Can you work these out from the model? Positions are in its coordinate system, mm. A direction names the side the tool comes from. Give positions to 0.01 mm unless a question says otherwise; leave off trailing zeros. Loops run counter-clockwise (first coordinate to the right, second up) from the corner with the lowest first, then second, coordinate; pieces in that order, holes last. Notation, with made-up numbers: (44.25, 35) -> (101.25, 35) arc R7 cw to (101.25, 46) -> close; hole circle Ø4 at (55, -11). An arc over 180 degrees is marked (long way). One line per question, with ' | ' between items.
from build123d import *

# Parameters (mm, degrees)
F0_W     = 101.6
F0_H     = 50.8
F1_DEPTH = 38.1


with BuildPart() as f1:
    # F0 (on Front) → F1 (new body, symmetric)
    with BuildSketch(Plane.XZ):
        with BuildLine():
            ThreePointArc((65.9712880145, -38.6489294899), (73.7903692418, -20.0232864477), (76.4588163197, 0))
            ThreePointArc((76.4588163197, 0), (73.9582301549, 19.3940915064), (66.6200350394, 37.5196151947))
            Line((66.6200350394, 37.5196151947), (65.9712880145, -38.6489294899))
        make_face()
        with BuildLine():
            Line((65.9712880145, -38.6489294899), (66.6200350394, 37.5196151947))
            ThreePointArc((66.6200350394, 37.5196151947), (66.5384735192, 37.6640695456), (66.4565987746, 37.808346596))
            Line((66.4565987746, 37.808346596), (0.8170776208, 76.4544503425))
            ThreePointArc((0.8170776208, 76.4544503425), (0.6511957232, 76.4560431695), (0.4853107601, 76.4572760859))
            Line((0.4853107601, 76.4572760859), (-65.8029574185, 38.9348351477))
            ThreePointArc((-65.8029574185, 38.9348351477), (-65.887277796, 38.7919736239), (-65.9712880145, 38.6489294899))
            Line((-65.9712880145, 38.6489294899), (-66.6200350394, -37.5196151947))
            ThreePointArc((-66.6200350394, -37.5196151947), (-66.5384735192, -37.6640695456), (-66.4565987746, -37.808346596))
            Line((-66.4565987746, -37.808346596), (-0.8170776208, -76.4544503425))
            ThreePointArc((-0.8170776208, -76.4544503425), (-0.6511957232, -76.4560431695), (-0.4853107601, -76.4572760859))
            Line((-0.4853107601, -76.4572760859), (65.8029574185, -38.9348351477))
            ThreePointArc((65.8029574185, -38.9348351477), (65.887277796, -38.7919736239), (65.9712880145, -38.6489294899))
        make_face()
        Rectangle(F0_W, F0_H, mode=Mode.SUBTRACT)
        with BuildLine():
            ThreePointArc((66.4565987746, 37.808346596), (66.5384735192, 37.6640695456), (66.6200350394, 37.5196151947))
            Line((66.6200350394, 37.5196151947), (66.6216664831, 37.7111608811))
            Line((66.6216664831, 37.7111608811), (66.4565987746, 37.808346596))
        make_face()
        with BuildLine():
            Line((65.9696565708, -38.8404751763), (65.9712880145, -38.6489294899))
            ThreePointArc((65.9712880145, -38.6489294899), (65.887277796, -38.7919736239), (65.8029574185, -38.9348351477))
            Line((65.8029574185, -38.9348351477), (65.9696565708, -38.8404751763))
        make_face()
        with BuildLine():
            Line((0.8170776208, 76.4544503425), (66.4565987746, 37.808346596))
            ThreePointArc((66.4565987746, 37.808346596), (38.7919736239, 65.887277796), (0.8170776208, 76.4544503425))
        make_face()
        with BuildLine():
            ThreePointArc((-0.4853107601, -76.4572760859), (37.6640695456, -66.5384735192), (65.8029574185, -38.9348351477))
            Line((65.8029574185, -38.9348351477), (-0.4853107601, -76.4572760859))
        make_face()
        with BuildLine():
            ThreePointArc((0.4853107601, 76.4572760859), (0.6511957232, 76.4560431695), (0.8170776208, 76.4544503425))
            Line((0.8170776208, 76.4544503425), (0.6520099123, 76.5516360573))
            Line((0.6520099123, 76.5516360573), (0.4853107601, 76.4572760859))
        make_face()
        with BuildLine():
            Line((-0.6520099123, -76.5516360573), (-0.4853107601, -76.4572760859))
            ThreePointArc((-0.4853107601, -76.4572760859), (-0.6511957232, -76.4560431695), (-0.8170776208, -76.4544503425))
            Line((-0.8170776208, -76.4544503425), (-0.6520099123, -76.5516360573))
        make_face()
        with BuildLine():
            Line((-65.8029574185, 38.9348351477), (0.4853107601, 76.4572760859))
            ThreePointArc((0.4853107601, 76.4572760859), (-37.6640695456, 66.5384735192), (-65.8029574185, 38.9348351477))
        make_face()
        with BuildLine():
            ThreePointArc((-66.4565987746, -37.808346596), (-38.7919736239, -65.887277796), (-0.8170776208, -76.4544503425))
            Line((-0.8170776208, -76.4544503425), (-66.4565987746, -37.808346596))
        make_face()
        with BuildLine():
            ThreePointArc((-65.9712880145, 38.6489294899), (-65.887277796, 38.7919736239), (-65.8029574185, 38.9348351477))
            Line((-65.8029574185, 38.9348351477), (-65.9696565708, 38.8404751763))
            Line((-65.9696565708, 38.8404751763), (-65.9712880145, 38.6489294899))
        make_face()
        with BuildLine():
            Line((-66.6216664831, -37.7111608811), (-66.4565987746, -37.808346596))
            ThreePointArc((-66.4565987746, -37.808346596), (-66.5384735192, -37.6640695456), (-66.6200350394, -37.5196151947))
            Line((-66.6200350394, -37.5196151947), (-66.6216664831, -37.7111608811))
        make_face()
        with BuildLine():
            Line((-66.6200350394, -37.5196151947), (-65.9712880145, 38.6489294899))
            ThreePointArc((-65.9712880145, 38.6489294899), (-76.4560431695, 0.6511957232), (-66.6200350394, -37.5196151947))
        make_face()
    extrude(amount=F1_DEPTH, both=True)


solid = f1.part
Q1. For pin 1 Ø10 at (y, z) = (14.5, -16.5) entering from +X; pin 2 Ø4 at (x, y) = (7, -15) entering from +Z; pin 3 Ø12 at (y, z) = (2.5, 5.5) entering from -X; pin 4 Ø6 at (x, y) = (-41.5, 28.5) entering from -Z, each with a flat end and sliding along its axis, tell me the tip position at first contact or that it passes through.
Entries:
pin 1: x = 75.59 | pin 2: z = 76.3 | pin 3: x = -76.46 | pin 4: z = -66.06
Q2. If we section it at C-C (z = -5): Write out the boundary of the cut face in (x, y).
Entries:
outline: (-76.3, -38.1) -> (-50.8, -38.1) -> (-50.8, 38.1) -> (-76.3, 38.1) -> close; (50.8, -38.1) -> (76.3, -38.1) -> (76.3, 38.1) -> (50.8, 38.1) -> close
Q3. If we section it at D-D (z = -27.5): Write out the boundary of the cut face in (x, y).
Entries:
outline: (-71.34, -38.1) -> (71.34, -38.1) -> (71.34, 38.1) -> (-71.34, 38.1) -> close
Q4. On a 3-axis mill with a long thin cutter (end or side, diameter ignored), from which of +Z, -Z, +X, -X, +Y, -Y can I reach the whole of each face in a straight line? I mean faces 1 (the face through (-1, -1, 25.4)), 2 (the face through (76.45, -0.53, -1.21)). Say none if no direction works.
Entries:
face 1: +Y, -Y | face 2: +X, +Y, -Y
Q5. If we mould it in two halves opening along X, with no side actions, what happens to faces 3 (the face through (-1, -38.1, -33)), 4 (the face through (-39.272, -0.533, -65.602)), 5 (the face through (-1, -1, -25.4))? For each: pulls with the +X half, pulls with the -X half, needs draft (parallel to the pull), parting line crosses it, or undercut.
Entries:
face 3: needs draft | face 4: pulls with the -X half | face 5: undercut
Q6. If I drill on probe 1 along Z at (x, y) = (32, 19); probe 2 along Z at (x, y) = (31, 1); probe 3 along X at (y, z) = (29.5, -1), over which ranges is the centre line in solid material (lowest first)? Write a range as from..to.
Entries:
probe 1: -69.44..-25.4, 25.4..69.44 | probe 2: -69.89..-25.4, 25.4..69.89 | probe 3: -76.45..-50.8, 50.8..76.45
Q7. If we section it at A-A (x = -4): Write out the boundary of the cut face in (y, z).
Entries:
outline: (-38.1, -76.35) -> (38.1, -76.35) -> (38.1, -25.4) -> (-38.1, -25.4) -> close; (-38.1, 25.4) -> (38.1, 25.4) -> (38.1, 76.35) -> (-38.1, 76.35) -> close
Q8. If we section it at B-B (y = 23): Write out the boundary of the cut face in (x, z).
Entries:
outline: (-66.62, -37.71) -> (-66.46, -37.81) arc R76.46 ccw to (-0.82, -76.45) -> (-0.65, -76.55) -> (-0.49, -76.46) arc R76.46 ccw to (65.8, -38.93) -> (65.97, -38.84) -> (65.97, -38.65) arc R76.46 ccw to (66.62, 37.52) -> (66.62, 37.71) -> (66.46, 37.81) arc R76.46 ccw to (0.82, 76.45) -> (0.65, 76.55) -> (0.49, 76.46) arc R76.46 ccw to (-65.8, 38.93) -> (-65.97, 38.84) -> (-65.97, 38.65) arc R76.46 ccw to (-66.62, -37.52) -> close; hole (-50.8, -25.4) -> (50.8, -25.4) -> (50.8, 25.4) -> (-50.8, 25.4) -> close
